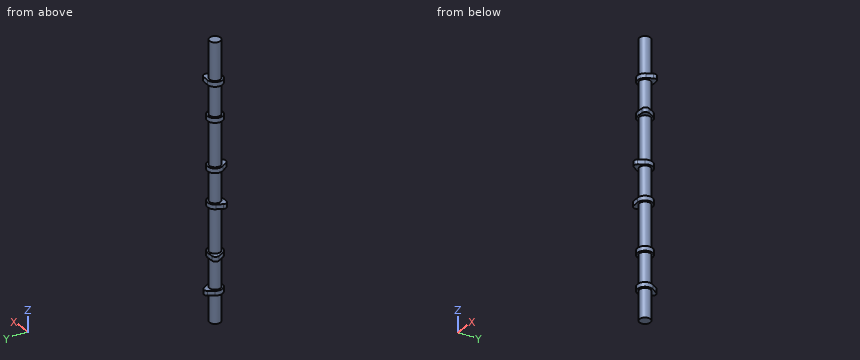
```python
from build123d import *

# Parameters (mm, degrees)
SKETCH1_R           = 9.5
BOSS_EXTRUDE1_DEPTH = 476
BOSS_EXTRUDE2_DEPTH = 8
BOSS_EXTRUDE3_DEPTH = 8
BOSS_EXTRUDE4_DEPTH = 8
BOSS_EXTRUDE5_DEPTH = 8
BOSS_EXTRUDE6_DEPTH = 8
BOSS_EXTRUDE7_DEPTH = 8


with BuildPart() as part:
    # Sketch1 → Boss-Extrude1 (new body)
    with BuildSketch(Plane.XY):
        Circle(SKETCH1_R)
    extrude(amount=BOSS_EXTRUDE1_DEPTH)

    # Sketch2 → Boss-Extrude2 (add)
    with BuildSketch(Plane(origin=(0, 0, 50), x_dir=(-1, 0, 0), z_dir=(0, 0, -1))):
        with BuildLine():
            Line((-10.954451152, 6.999999997), (-5.055900535, 16.230769231))
            ThreePointArc((-5.055900535, 16.230769231), (-1e-09, 19.000000003), (5.055900534, 16.230769233))
            Line((5.055900534, 16.230769233), (10.954451152, 6.999999997))
            ThreePointArc((10.954451152, 6.999999997), (0, -13), (-10.954451152, 6.999999997))
        make_face()
    extrude(amount=-BOSS_EXTRUDE2_DEPTH)

    # Sketch3 → Boss-Extrude3 (add)
    with BuildSketch(Plane.XY.offset(111)):
        with BuildLine():
            Line((-0.584952247, 12.986832981), (-11.52830821, 12.493922918))
            ThreePointArc((-11.52830821, 12.493922918), (-16.454482674, 9.500000003), (-16.584208745, 3.736846315))
            Line((-16.584208745, 3.736846315), (-11.5394034, -5.986832984))
            ThreePointArc((-11.5394034, -5.986832984), (11.258330249, -6.5), (-0.584952247, 12.986832981))
        make_face()
    extrude(amount=BOSS_EXTRUDE3_DEPTH)

    # Sketch4 → Boss-Extrude4 (add)
    with BuildSketch(Plane.XY.offset(196)):
        with BuildLine():
            Line((-11.5394034, 5.986832984), (-16.584208744, -3.736846313))
            ThreePointArc((-16.584208744, -3.736846313), (-16.454482675, -9.500000001), (-11.528308212, -12.493922917))
            Line((-11.528308212, -12.493922917), (-0.584952247, -12.986832981))
            ThreePointArc((-0.584952247, -12.986832981), (11.258330249, 6.5), (-11.5394034, 5.986832984))
        make_face()
    extrude(amount=BOSS_EXTRUDE4_DEPTH)

    # Sketch5 → Boss-Extrude5 (add)
    with BuildSketch(Plane.XY.offset(257)):
        with BuildLine():
            Line((-10.954451152, -6.999999997), (-5.055900535, -16.230769231))
            ThreePointArc((-5.055900535, -16.230769231), (-1e-09, -19.000000003), (5.055900534, -16.230769233))
            Line((5.055900534, -16.230769233), (10.954451152, -6.999999997))
            ThreePointArc((10.954451152, -6.999999997), (0, 13), (-10.954451152, -6.999999997))
        make_face()
    extrude(amount=BOSS_EXTRUDE5_DEPTH)

    # Sketch6 → Boss-Extrude6 (add)
    with BuildSketch(Plane.XY.offset(342)):
        with BuildLine():
            Line((0.584952247, -12.986832981), (11.52830821, -12.493922918))
            ThreePointArc((11.52830821, -12.493922918), (16.454482674, -9.500000003), (16.584208745, -3.736846315))
            Line((16.584208745, -3.736846315), (11.5394034, 5.986832984))
            ThreePointArc((11.5394034, 5.986832984), (-11.258330249, 6.5), (0.584952247, -12.986832981))
        make_face()
    extrude(amount=BOSS_EXTRUDE6_DEPTH)

    # Sketch7 → Boss-Extrude7 (add)
    with BuildSketch(Plane.XY.offset(403)):
        with BuildLine():
            Line((11.5394034, -5.986832984), (16.584208744, 3.736846313))
            ThreePointArc((16.584208744, 3.736846313), (16.454482675, 9.500000001), (11.528308212, 12.493922917))
            Line((11.528308212, 12.493922917), (0.584952247, 12.986832981))
            ThreePointArc((0.584952247, 12.986832981), (-11.258330249, -6.5), (11.5394034, -5.986832984))
        make_face()
    extrude(amount=BOSS_EXTRUDE7_DEPTH)


solid = part.part
```
Check sheet for the modelled part. Datum: model origin and axes. Units: mm. Give positions to 0.01 mm unless a question says otherwise; leave off trailing zeros. Loops run counter-clockwise (first coordinate to the right, second up) from the corner with the lowest first, then second, coordinate; pieces in that order, holes last. Notation, with made-up numbers: (38.5, 48.25) - (60.5, 48.25) arc R20 cw to (60.5, 58.25) - close; hole circle Ø6 at (52, -23.75). An arc over 180 degrees is marked (long way). One line per question, with ' | ' between items. Start each with the question number.
1. Gauge pin test, flat ends, axial feed: pin 1 Ø12 at (y, z) = (0.5, 191.5) entering from +X; pin 2 Ø1.5 at (x, z) = (-9.5, 414.5) entering from -Y; pin 3 Ø1.5 at (x, z) = (3, 112) entering from +Y. Record the tip position at first contact, or that the pin passes through.
2. Material ranges on line 1 along Z through (x, y) = (-10.5, -2.5); line 2 along Z through (x, y) = (-1, 13); line 3 along Z through (x, y) = (-16, -3.5), recorded low to high. Write a range as [from, to].
3. Cross-section at A-A, the plane z = 235. Enter the section's corners in (x, y), plus the area to 3 significant figures.
Check result:
1) pin 1: stops at x = 13 | pin 2: stops at y = -3.7 | pin 3: stops at y = 12.8
2) line 1: z = [50, 58], [111, 119], [196, 204], [257, 265], [342, 350], [403, 411] | line 2: z = [50, 58] | line 3: z = [196, 204]
3) outline: circle Ø19 at (0, 0) | area: 284 mm2
